Here's how the part is built. I have some questions about the finished solid (model axes, mm). Coordinates: 2 decimals unless noted, no trailing zeros. Order: outer loops, then holes, each group sorted by start corner. A loop starts at its lowest first (then second) coordinate and runs counter-clockwise, first axis right, second up.
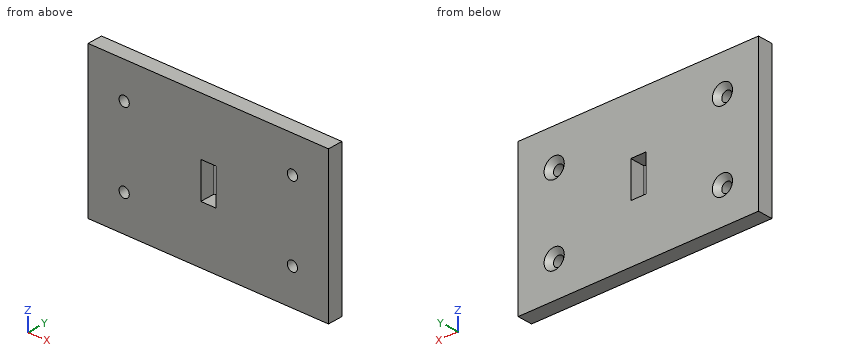
```python
from build123d import *

# Parameters (mm, degrees)
SKETCH1_W                                            = 80
SKETCH1_H                                            = 50
BOSS_EXTRUDE1_DEPTH                                  = 2.5
SKETCH2_W                                            = 5
SKETCH2_H                                            = 12
CUT_EXTRUDE1_DEPTH                                   = 5
CSK_FOR_M3_HEX_SOCKET_COUNTERSUNK_CAP_SC_D           = 3.4
CSK_FOR_M3_HEX_SOCKET_COUNTERSUNK_CAP_SC_CSINK_D     = 6.72
CSK_FOR_M3_HEX_SOCKET_COUNTERSUNK_CAP_SC_CSINK_ANGLE = 90


with BuildPart() as part:
    # Sketch1 → Boss-Extrude1 (new, symmetric)
    with BuildSketch(Plane(origin=(0, 0, 0), x_dir=(1, 0, 0), z_dir=(0, 1, 0))):
        Rectangle(SKETCH1_W, SKETCH1_H)
    extrude(amount=BOSS_EXTRUDE1_DEPTH, both=True)

    # Sketch2 → Cut-Extrude1 (cut)
    with BuildSketch(Plane(origin=(0, 2.5, 0), x_dir=(1, 0, 0), z_dir=(0, 1, 0))):
        Rectangle(SKETCH2_W, SKETCH2_H)
    extrude(amount=-CUT_EXTRUDE1_DEPTH, mode=Mode.SUBTRACT)

    # CSK for M3 Hex Socket Countersunk Cap Screw1 (through all)
    with Locations(Plane(origin=(0, 2.5, 0), x_dir=(1, 0, 0), z_dir=(0, 1, 0))):
        with Locations((28, -13), (28, 13), (-28, -13), (-28, 13)):
            CounterSinkHole(CSK_FOR_M3_HEX_SOCKET_COUNTERSUNK_CAP_SC_D / 2, CSK_FOR_M3_HEX_SOCKET_COUNTERSUNK_CAP_SC_CSINK_D / 2, counter_sink_angle=CSK_FOR_M3_HEX_SOCKET_COUNTERSUNK_CAP_SC_CSINK_ANGLE)


solid = part.part
```
Q1. If we section it at B-B on z = 13: Write out the boundary of the cut face in (x, y).
Q2. If we section it at D-D on x = -28: Write out the boundary of the cut face in (y, z), then the cut area to 3 significant figures.
Q3. Will these pins go through, and if not, where does the flat tip stop? pin 1 (4 mm diameter, centred on x = 28, z = 13, fed in from +Y); pin 2 (4.5 mm diameter, centred on x = -28, z = 13, fed in from +Y).
Q4. If we section it at A-A on y = -0.25: Write out the boundary of the cut face in (x, z).
Q5. I need wall thicknesses on L1, parallel to Z at x = -28, y = -0.3; L2, parallel to X at y = -1.5, z = 13; L3, parallel to X at y = 0.3, z = 2. Which ranges of each line are inside material? Lowest first, please.
Q6. If we section it at C-C on x = -0.5: Write out the boundary of the cut face in (y, z), then the cut area to 3 significant figures.
Reply:
1. outline: (-40, -2.5) - (-29.7, -2.5) - (-29.7, 0.84) - (-31.36, 2.5) - (-40, 2.5) - close; (-26.3, -2.5) - (26.3, -2.5) - (26.3, 0.84) - (24.64, 2.5) - (-24.64, 2.5) - (-26.3, 0.84) - close; (29.7, -2.5) - (40, -2.5) - (40, 2.5) - (31.36, 2.5) - (29.7, 0.84) - close
2. outline: (-2.5, -25) - (2.5, -25) - (2.5, -16.36) - (0.84, -14.7) - (-2.5, -14.7) - close; (-2.5, -11.3) - (0.84, -11.3) - (2.5, -9.64) - (2.5, 9.64) - (0.84, 11.3) - (-2.5, 11.3) - close; (-2.5, 14.7) - (0.84, 14.7) - (2.5, 16.36) - (2.5, 25) - (-2.5, 25) - close
2. area: 210 mm2
3. pin 1: stops at y = 1.14
3. pin 2: stops at y = 1.39
4. outline: (-40, -25) - (40, -25) - (40, 25) - (-40, 25) - close; hole circle Ø3.4 at (-28, -13); hole circle Ø3.4 at (-28, 13); hole (-2.5, -6) - (2.5, -6) - (2.5, 6) - (-2.5, 6) - close; hole circle Ø3.4 at (28, -13); hole circle Ø3.4 at (28, 13)
5. L1: z = -25 to -14.7, -11.3 to 11.3, 14.7 to 25
5. L2: x = -40 to -29.7, -26.3 to 26.3, 29.7 to 40
5. L3: x = -40 to -2.5, 2.5 to 40
6. outline: (-2.5, -25) - (2.5, -25) - (2.5, -6) - (-2.5, -6) - close; (-2.5, 6) - (2.5, 6) - (2.5, 25) - (-2.5, 25) - close
6. area: 190 mm2
